Input: part model. Units: mm. Frame: model coordinates. Round coordinates to 2 decimals unless told otherwise and drop trailing zeros. Order: outer loops, then holes, each group sorted by start corner. A loop starts at its lowest first (then second) coordinate and runs counter-clockwise, first axis right, second up. Notation, with made-up numbers: M 39.25,48.25 L 76.25,48.25 A35 ccw 76.25,82.25 Z; hole C -12.5,-14 d8. An arc over 180 degrees is marked long. One line per question, with ' | ' between items.
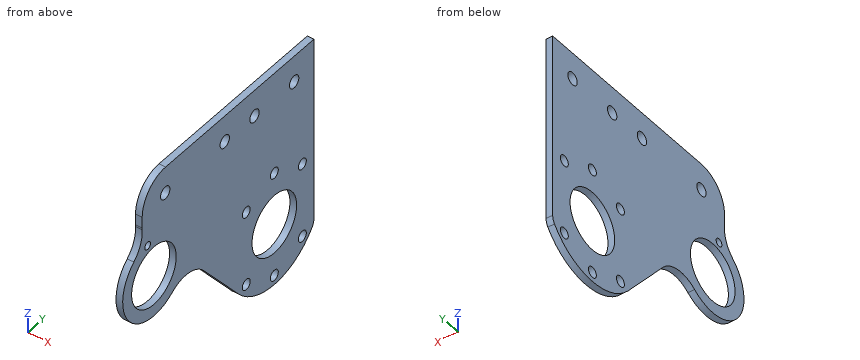
Autodesk Inventor part; units mm, degrees
ref_plane "YZ Plane" through (0, 0, 0) normal (1, 0, 0) x (0, 1, 0)
ref_plane "XZ Plane" through (0, 0, 0) normal (0, 1, 0) x (-1, 0, 0)
ref_plane "XY Plane" through (0, 0, 0) normal (0, 0, 1) x (1, 0, 0)
sketch "Sketch1" plane through (0, 0, 0) normal (1, 0, 0) x (0, 1, 0)
  line L0 (-39.3892, -105) -> (-110, -20.8494)
  line L1 (-110, -20.8494) -> (-110, 0)
  line L2 (-110, 0) -> (0, 0)
  line L3 (0, 0) -> (0, -105)
  line L4 (0, -105) -> (-39.3892, -105)
  line L5 (-110, -20.8494) -> (-119.38, 0) construction
  line L6 (-119.38, 0) -> (-110, 0) construction
  line L7 (-50.8, -25.4) -> (0, -25.4) construction
  line L8 (0, -25.4) -> (0, 0) construction
  line L9 (0, 0) -> (-50.8, 0) construction
  line L10 (-50.8, 0) -> (-50.8, -25.4) construction
  line L11 (-50.8, -25.4) -> (0, 0) construction
  line L12 (0, -25.4) -> (-50.8, 0) construction
  circle A0 centre (-12.7, -12.7) radius 3
  circle A1 centre (-38.1, -12.7) radius 3
  circle A2 centre (-102.5, -49) radius 14.2875
  circle A3 centre (-25.4, -75) radius 14.2875
  circle A4 centre (-102.5, -49) radius 20
  circle A5 centre (-25.4, -75) radius 30
  line L13 (-50.8, -90.9637) -> (-50.8, -59.0363)
  line L14 (-102.5, -49) -> (-25.4, -75) construction
  circle A6 centre (-57.15, -12.7) radius 3
  circle A7 centre (-95.25, -12.7) radius 3
  point P0 (-25.4, -12.7)
  point P1 (-25.4, -25.4)
  point P2 (-103.1519, -29.0106)
  point P3 (-82.9275, -53.1131)
  point P4 (-50.8, -75)
  point P5 (-48.3813, -94.2836)
  point P6 (0, -90.9637)
  dimension "d0" = 50
  dimension "d1" = 119.38
  dimension "d2" = 50.8
  dimension "d3" = 25.4
  dimension "d4" = 25.4
  dimension "d5" = 12.7
  dimension "d6" = 6
  dimension "d7" = 6
  dimension "d8" = 28.575
  dimension "d9" = 102.5
  dimension "d10" = 49
  dimension "d13" = 110
  dimension "d16" = 60
  dimension "d17" = 25.4
  dimension "d18" = 25.4
  dimension "d20" = 40
  dimension "d44" = 81.3659
  dimension "d45" = 38.1
  dimension "d46" = 19.05
extrude "Plate1" add sketch "Sketch1" along normal blind 3.175 contours L0 A4 L1 L2 L3 A5 | A5 L13 L3 | A4 L0 A2 | L0 A2 A4 | A5 L13
fillet "Corner Round1" radius 15 4 edges at (1.5875, -82.9275, -53.1131) (1.5875, -103.1519, -29.0106) (1.5875, -110, -20.8494) (1.5875, -110, 0)
fillet "Corner Round1" radius 6 1 edges at (1.5875, 0, -90.9637)
sketch "Sketch2" plane through (0, 0, 0) normal (-1, 0, 0) x (0, 0, 1)
  circle A0 centre (-31.4501, -106.5) radius 4.5847
  circle A1 centre (-49, -102.5) radius 14.2875
  point P0 (0, 0)
  dimension "d21" = 9.1694
  dimension "d22" = 18
  dimension "d23" = 4
hole "Hole1" at (0, -106.5, -31.4501) direction (1, 0, 0) diameter 3.683 end through all
sketch "Sketch3" plane through (3.175, 0, 0) normal (1, 0, 0) x (0, 0, -1)
  circle A0 centre (75, -25.4) radius 14.2875
  circle A1 centre (75, -25.4) radius 25.4
  line L0 (49.6, -25.4) -> (100.4, -25.4)
  line L1 (92.9605, -7.4395) -> (57.0395, -7.4395)
  line L2 (75, -25.4) -> (57.0395, -7.4395)
  line L3 (92.9605, -43.3605) -> (57.0395, -43.3605)
  line L4 (75, -25.4) -> (92.9605, -43.3605)
  line L5 (25.4, -50.8) -> (0, -50.8)
  line L6 (0, -50.8) -> (0, 0)
  line L7 (0, 0) -> (25.4, 0)
  line L8 (25.4, 0) -> (25.4, -50.8)
  line L9 (25.4, -50.8) -> (0, 0) construction
  line L10 (0, -50.8) -> (25.4, 0) construction
  point P0 (12.7, -25.4)
  dimension "d31" = 50.8
  dimension "d32" = 45
  dimension "d40" = 25.4
  dimension "d41" = 50.8
hole "Hole2" at (3.175, -7.4395, -57.0395) at (3.175, -25.4, -49.6) at (3.175, -43.3605, -57.0395) at (3.175, -43.3605, -92.9605) at (3.175, -25.4, -100.4) at (3.175, -7.4395, -92.9605) direction (-1, 0, 0) diameter 5.105 end through all
equation "\"d7\" = d6"
equation "\"d29\" = Thickness"
equation "\"d14\" = Thickness"
equation "\"BendRadius\" = Thickness"
equation "\"BendReliefWidth\" = Thickness"
equation "\"BendReliefDepth\" = 0.5 * Thickness"
equation "\"CornerReliefSize\" = 4 * Thickness"
equation "\"MinimumRemnant\" = 2 * Thickness"
equation "\"TransitionRadius\" = BendRadius"
equation "\"JacobiRadiusSize\" = BendRadius"
equation "\"GapSize\" = Thickness"
properties part number "INSIDE_INTAKE_PLATE" material "Aluminum, 6061-T6"
Item 1: Line query: line 1 along Z through (x, y) = (0.55, -45); line 2 along Z through (x, y) = (3.05, -44); line 3 along Y through (x, z) = (1.4, -94.5). Output: solid intervals per line, ascending. Write a range as from..to.
Report:
line 1: -97.71..-94.92, -91..-59, -55.08..0 | line 2: -98.54..-95.43, -90.49..-59.51, -54.57..0 | line 3: -48.2..-45.4, -41.32..-9.48, -5.4..-2.6
Item 2: Section query B-B, the plane y = -12.7. Return loops of the section in (x, z) (3 decimals).
Report:
outline: M 0,-102.179 L 3.175,-102.179 L 3.175,-81.545 L 0,-81.545 Z; M 0,-68.455 L 3.175,-68.455 L 3.175,-15.7 L 0,-15.7 Z; M 0,-9.7 L 3.175,-9.7 L 3.175,0 L 0,0 Z
Item 3: Section query A-A, the plane z = -12.7. Return loops of the section in (x, y) (3 decimals), plus the area to 3 significant figures.
Report:
outline: M 0,-109.823 L 3.175,-109.823 L 3.175,-98.25 L 0,-98.25 Z; M 0,-92.25 L 3.175,-92.25 L 3.175,-60.15 L 0,-60.15 Z; M 0,-54.15 L 3.175,-54.15 L 3.175,-41.1 L 0,-41.1 Z; M 0,-35.1 L 3.175,-35.1 L 3.175,-15.7 L 0,-15.7 Z; M 0,-9.7 L 3.175,-9.7 L 3.175,0 L 0,0 Z | area: 272 mm²
Item 4: Section query C-C, the plane z = -44. Return loops of the section in (x, y) (3 decimals).
Report:
outline: M 0,-121.865 L 3.175,-121.865 L 3.175,-115.884 L 0,-115.884 Z; M 0,-89.116 L 3.175,-89.116 L 3.175,0 L 0,0 Z
Item 5: Section query D-D, the plane x = 1.75. Give the number of separate pieces and of enclosed holes in the cut face, plus the area to 3 significant figures.
Report:
separate pieces: 1 | enclosed holes: 13 | area: 8,060 mm²
Item 6: First-contact query: pin 1 (1.6 mm diameter, centred on x = 1.5, z = -17.5, fed in from -Y); pin 2 (1.5 mm diameter, centred on x = 1.5, y = -20.5, fed in from -Z). Flat tips, straight axial feed; report the tip coordinate or a pass-through.
Report:
pin 1: y = -110 | pin 2: z = -104.71
